Autodesk Inventor part; units mm, degrees
ref_plane "YZ Plane" through (0, 0, 0) normal (1, 0, 0) x (0, 1, 0)
ref_plane "XZ Plane" through (0, 0, 0) normal (0, 1, 0) x (-1, 0, 0)
ref_plane "XY Plane" through (0, 0, 0) normal (0, 0, 1) x (1, 0, 0)
sketch "本体面" plane through (0, 0, 0) normal (0, 0, 1) x (1, 0, 0)
  line L0 (-18.8, 10) -> (18.8, 10)
  line L1 (18.8, 10) -> (18.8, 0)
  line L2 (18.8, 0) -> (-18.8, 0)
  line L3 (-18.8, 0) -> (-18.8, 10)
  point P0 (0, 0)
  point P1 (0, 0)
  dimension "d0" = 37.6
  dimension "d1" = 10
extrude "本体" add sketch "本体面" along normal blind 44
sketch "空洞面" plane through (0, 0, 44) normal (0, 0, 1) x (1, 0, 0)
  line L0 (-17, 10) -> (17, 10)
  line L1 (17, 10) -> (17, 3)
  line L2 (15, 1) -> (-15, 1)
  line L3 (-17, 3) -> (-17, 10)
  line L4 (18.8, 10) -> (-18.8, 10)
  arc A0 (-17, 3) -> (-15, 1) centre (-15, 3) ccw
  arc A1 (15, 1) -> (17, 3) centre (15, 3) ccw
  point P0 (0, 0)
  point P1 (17, 1)
  point P2 (-17, 1)
  point P3 (0, 10)
  dimension "d4" = 34
  dimension "d5" = 9
  dimension "d6" = 2
extrude "空洞" cut sketch "空洞面" against normal up to surface (44 mm away)
sketch "溝形状" plane through (0, 0, 44) normal (0, 0, 1) x (1, 0, 0)
  line L0 (-17, 10) -> (-18.8, 10) construction
  line L1 (-18.8, 10) -> (-18.8, 0) construction
  line L2 (-17, 3) -> (-17, 10) construction
  line L3 (17, 9.6) -> (-17, 9.6)
  line L4 (-17, 9.6) -> (-18, 8.6)
  line L5 (18, 8.6) -> (17, 9.6)
  line L6 (18.8, 0) -> (18.8, 10) construction
  line L7 (18.8, 10) -> (17, 10) construction
  line L8 (17, 10) -> (17, 3) construction
  line L9 (-18, 8.6) -> (-18, 7)
  line L10 (-18, 7) -> (18, 7)
  line L11 (18, 7) -> (18, 8.6)
  line L12 (-10, 9) -> (10, 9) construction
  line L13 (10, 9) -> (10, 7) construction
  line L14 (10, 7) -> (-10, 7) construction
  line L15 (-10, 7) -> (-10, 9) construction
  point P0 (0, 0)
  point P1 (0, 7)
  dimension "d31" = 135
  dimension "d34" = 0.8
  dimension "d35" = 0.4
  dimension "d36" = 0.8
  dimension "d37" = 135
  dimension "d38" = 2.6
  dimension "d41" = 2
  dimension "d42" = 20
extrude "溝" cut sketch "溝形状" against normal blind 43
sketch "底中央" plane through (-18.8, 0, 0) normal (0, -1, 0) x (1, 0, 0)
  line L0 (0, 0) -> (0, 44) construction
  line L1 (37.6, 0) -> (0, 0) construction
  point P0 (18.8, 0)
  point P1 (18.8, 22)
  point P2 (0, 22)
  point P3 (18.8, 0)
sketch "スケッチ8" plane through (-15, 1, 44) normal (0, 1, 0) x (1, 0, 0)
  line L0 (30, 0) -> (30, 44)
  line L1 (-2, 44) -> (0, 44)
  line L2 (0, 0) -> (0, 44)
  line L3 (30, 44) -> (32, 44)
  circle A0 centre (15, 22) radius 1.5
  point P0 (15, 44)
  dimension "d50" = 3
extrude "押し出し5" cut sketch "スケッチ8" against normal through all
properties part number "HB5_holder"
Could you check a few things on this model? Use its own coordinates, in mm. A direction names the side the tool comes from. Coordinates: 2 decimals unless noted, no trailing zeros. Order: outer loops, then holes, each group sorted by start corner. A loop starts at its lowest first (then second) coordinate and runs counter-clockwise, first axis right, second up. Notation, with made-up numbers: (-17.5, 50.25) -> (-4.5, 50.25) arc R33 ccw to (-4.5, 88.25) -> close; hole circle Ø1 at (-28, 71). An arc over 180 degrees is marked (long way). One line per question, with ' | ' between items.
Q1. Imagine slicing it at D-D on z = 17.5. Please give me the cut outline in (x, y).
Return value:
outline: (-18.8, 0) -> (18.8, 0) -> (18.8, 10) -> (17, 10) -> (17, 9.6) -> (18, 8.6) -> (18, 7) -> (17, 7) -> (17, 3) arc R2 cw to (15, 1) -> (-15, 1) arc R2 cw to (-17, 3) -> (-17, 7) -> (-18, 7) -> (-18, 8.6) -> (-17, 9.6) -> (-17, 10) -> (-18.8, 10) -> close
Q2. I'm going to push flat-ended pins straight in: P1, Ø6, axis at x = -3, y = 5, coming from the +Z side; P2, Ø9, axis at x = -7, z = 12.5, coming from the +Y side; P3, Ø0.5, axis at x = 17.5, y = 7.5, coming from the +Z side. Where does each tip first touch, or does it pass through?
Return value:
P1: through | P2: y = 1 | P3: z = 1
Q3. If I drill on L1, parallel to Z at x = 0, y = 0.3; L2, parallel to X at y = 8.5, z = 17; L3, parallel to X at y = 0.6, z = 22, over which ranges is the centre line in solid material (lowest first)?
Return value:
L1: 0 to 20.5, 23.5 to 44 | L2: -18.8 to -18, 18 to 18.8 | L3: -18.8 to -1.5, 1.5 to 18.8
Q4. Imagine slicing it at B-B on z = 22. Please give me the cut outline in (x, y).
Return value:
outline: (-18.8, 0) -> (-1.5, 0) -> (-1.5, 1) -> (-15, 1) arc R2 cw to (-17, 3) -> (-17, 7) -> (-18, 7) -> (-18, 8.6) -> (-17, 9.6) -> (-17, 10) -> (-18.8, 10) -> close; (1.5, 0) -> (18.8, 0) -> (18.8, 10) -> (17, 10) -> (17, 9.6) -> (18, 8.6) -> (18, 7) -> (17, 7) -> (17, 3) arc R2 cw to (15, 1) -> (1.5, 1) -> close
Q5. Imagine slicing it at C-C on x = 0. Please give me the cut outline in (y, z), and give its area (3 significant figures).
Return value:
outline: (0, 0) -> (1, 0) -> (1, 20.5) -> (0, 20.5) -> close; (0, 23.5) -> (1, 23.5) -> (1, 44) -> (0, 44) -> close | area: 41.0 mm²
Q6. Imagine slicing it at A-A on y = 6.5. Please give me the cut outline in (x, z).
Return value:
outline: (-18.8, 0) -> (-17, 0) -> (-17, 44) -> (-18.8, 44) -> close; (17, 0) -> (18.8, 0) -> (18.8, 44) -> (17, 44) -> close
Q7. On a 3-axis mill with a long thin cutter (end or side, diameter ignored), from which of +Z, -Z, +X, -X, +Y, -Y can I reach the whole of each face in a straight line? I mean faces 4 (the face through (17.5, 9.1, 22.8)), 5 (the face through (-0.195, 0.507, 20.513)), 6 (the face through (-16.43, 1.6, 22.31)). Say none if no direction works.
Return value:
face 4: +Z | face 5: +Y, -Y | face 6: +Z, -Z, +Y
Q8. Thinking about a two-plate mould opening in X: for faces 1 (the face through (4, 0, 22)), 2 (the face through (18.8, 5, 22)), 3 (the face through (17.5, 7, 22.8)), which applies, pulls with the +X half, pulls with the -X half, needs draft (parallel to the pull), parting line crosses it, or undercut?
Return value:
face 1: needs draft | face 2: pulls with the +X half | face 3: undercut
